Job drawing, mm, ordinate dimensions from the low corner. One solid piece. Coordinates: 2 decimals unless noted, no trailing zeros. Order: outer loops, then holes, each group sorted by start corner. A loop starts at its lowest first (then second) coordinate and runs counter-clockwise, first axis right, second up. Notation, with made-up numbers: (17.5, 78) - (66.5, 78) arc R23 ccw to (66.5, 108) - close; hole circle Ø9 at (-30.5, 77.5). An arc over 180 degrees is marked (long way). Use a Markdown table: item, result. Add a question column.
1) Wall check: L1, parallel to Y at x = 20, z = 3.6; L2, parallel to X at y = 13, z = 9.75; L3, parallel to Z at x = 19, y = 12.5. Give the ranges that are in metal, low to high. Write a range as [from, to].
2) Saw through at A-A on x = 20. List the corners of the cut face in (y, z), then the cut area to 4 significant figures.
3) Saw through at C-C on z = 12. List the corners of the cut face in (x, y).
4) Saw through at B-B on y = 15. List the corners of the cut face in (x, z).
5) Drop flat-ended pins along their axis: P1, Ø5, axis at x = 20, y = 15, coming from the +Z side; P2, Ø1.8, axis at x = 19.5, y = 14.5, coming from the +Z side; P3, Ø5, axis at x = 81.5, z = 21, coming from the -Y side; P4, Ø6.5, axis at x = 100.5, y = 15, coming from the +Z side. Give the stop position or say it passes through.
6) Saw through at D-D on z = 27.5. List the corners of the cut face in (x, y), then the cut area to 3 significant figures.
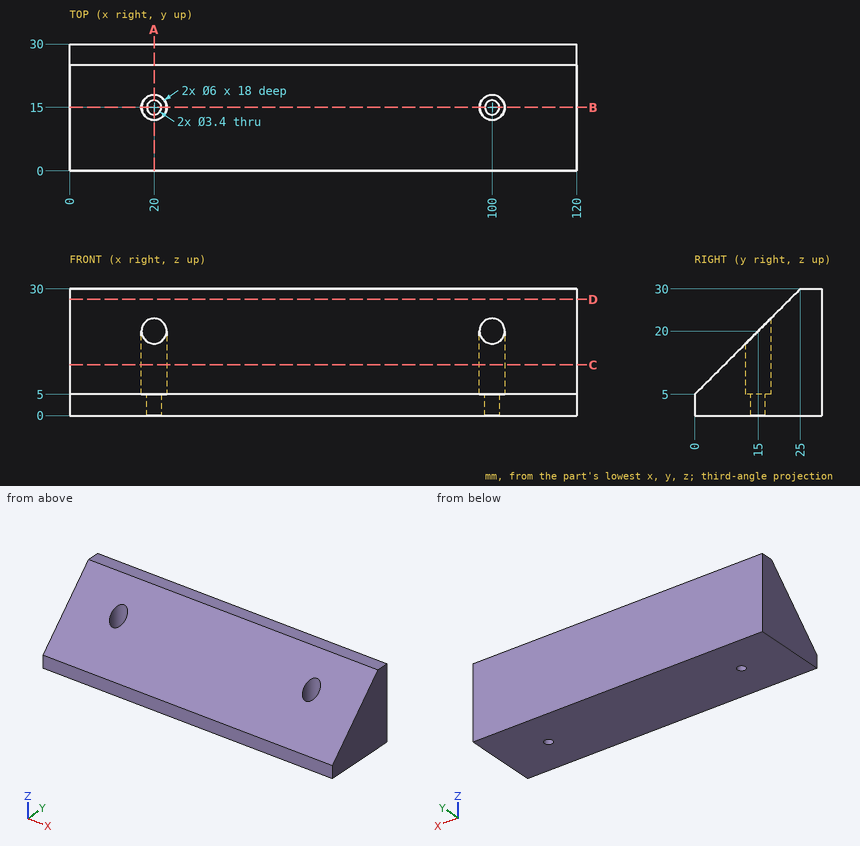
Results are:
| question | item | result |
|---|---|---|
| 1 | L1 | [0, 13.3], [16.7, 30] |
| 1 | L2 | [0, 17.76], [22.24, 97.76], [102.24, 120] |
| 1 | L3 | [0, 5] |
| 2 | outline | (0, 0) - (13.3, 0) - (13.3, 5) - (12, 5) - (12, 17) - (0, 5) - close; (16.7, 0) - (30, 0) - (30, 30) - (25, 30) - (18, 23) - (18, 5) - (16.7, 5) - close |
| 2 | area | 480.5 mm2 |
| 3 | outline | (0, 7) - (120, 7) - (120, 30) - (0, 30) - close; hole circle Ø6 at (20, 15); hole circle Ø6 at (100, 15) |
| 4 | outline | (0, 0) - (18.3, 0) - (18.3, 5) - (17, 5) - (17, 20) - (0, 20) - close; (21.7, 0) - (98.3, 0) - (98.3, 5) - (97, 5) - (97, 20) - (23, 20) - (23, 5) - (21.7, 5) - close; (101.7, 0) - (120, 0) - (120, 20) - (103, 20) - (103, 5) - (101.7, 5) - close |
| 5 | P1 | z = 5 |
| 5 | P2 | through |
| 5 | P3 | y = 13.5 |
| 5 | P4 | z = 23.25 |
| 6 | outline | (0, 22.5) - (120, 22.5) - (120, 30) - (0, 30) - close |
| 6 | area | 900 mm2 |
